from build123d import *

# Parameters (mm, degrees)
PAD_DEPTH            = 70
SKETCH001_W          = 11.887794
SKETCH001_H          = 46.78
POCKET_DEPTH         = 70.001
POCKET001_DEPTH      = 30
SKETCH003_R          = 2.5
POCKET002_DEPTH      = 40.001
SKETCH004_W          = 17
SKETCH004_H          = 23.314381
POCKET003_DEPTH      = 40.001
SKETCH005_W          = 35
SKETCH005_H          = 57.974789
POCKET004_DEPTH      = 26
SKETCH006_W          = 45.255611
SKETCH006_H          = 30.428207
POCKET005_DEPTH      = 28
POCKET005_DEPTH_BACK = -100
SKETCH007_W          = 26.242121
SKETCH007_H          = 29.741062
POCKET006_DEPTH      = 45
SKETCH008_W          = 15.625622
SKETCH008_H          = 14.392597
SKETCH008_W_2        = 24.610352
SKETCH008_H_2        = 31.67345
POCKET007_DEPTH      = 45
SKETCH009_R          = 2.5
POCKET008_DEPTH      = 13
SKETCH010_R          = 1.6
POCKET009_DEPTH      = 5
SKETCH014_W          = 10
SKETCH014_H          = 15
PAD001_DEPTH         = 23
SKETCH015_W          = 11
SKETCH015_H          = 38.184422
SKETCH015_W_2        = 19.881198
SKETCH015_H_2        = 10
PAD002_DEPTH         = 8
SKETCH013_R          = 2.5
POCKET010_DEPTH      = 17
SKETCH011_R          = 2.5
POCKET011_DEPTH      = 15
PAD003_DEPTH         = 5
SKETCH017_R          = 3
POCKET012_DEPTH      = 2
FILLET_R             = 1
FILLET001_R          = 7
FILLET002_R          = 1
FILLET003_R          = 1
FILLET004_R          = 2
FILLET005_R          = 2
FILLET006_R          = 18


with BuildPart() as part:
    # Sketch → Pad (new body)
    with BuildSketch(Plane.XY):
        Polygon((0, 0), (45, 0), (45, -50), (-28, -50), (-28, 0), align=None)
    extrude(amount=PAD_DEPTH)

    # Sketch001 (on Face7 of Pad) → Pocket (cut, through all)
    with BuildSketch(Plane.XY.offset(70)):
        with Locations((34.056103, -28.39)):
            Rectangle(SKETCH001_W, SKETCH001_H)
    extrude(amount=-POCKET_DEPTH, mode=Mode.SUBTRACT)

    # Sketch002 (on Face5 of Pocket) → Pocket001 (cut)
    with BuildSketch(Plane.XY.offset(70)):
        Polygon((30, -5), (30, -65.096024), (-40.783405, -65.096024), (-40.783405, 12.994774), (20, 12.994774), (20, -5), align=None)
    extrude(amount=-POCKET001_DEPTH, mode=Mode.SUBTRACT)

    # Sketch003 (on Face6 of Pocket001) → Pocket002 (cut, through all)
    with BuildSketch(Plane.XY.offset(40)):
        with Locations((-22, -40)):
            Circle(SKETCH003_R)
        with Locations((22, -40)):
            Circle(SKETCH003_R)
    extrude(amount=-POCKET002_DEPTH, mode=Mode.SUBTRACT)

    # Sketch004 (on Face6 of Pocket002) → Pocket003 (cut, through all)
    with BuildSketch(Plane.XY.offset(40)):
        with Locations((0, -43.65719)):
            Rectangle(SKETCH004_W, SKETCH004_H)
    extrude(amount=-POCKET003_DEPTH, mode=Mode.SUBTRACT)

    # Sketch005 (on Face13 of Pocket003) → Pocket004 (cut)
    with BuildSketch(Plane.XZ.offset(50)):
        with Locations((0, 7.512606)):
            Rectangle(SKETCH005_W, SKETCH005_H)
    extrude(amount=-POCKET004_DEPTH, mode=Mode.SUBTRACT)

    # Sketch006 (on Face11 of Pocket004) → Pocket005 (cut, two sides)
    with BuildSketch(Plane.XZ.offset(24)) as pocket005_sk:
        with Locations((-10.127806, 6.785896)):
            Rectangle(SKETCH006_W, SKETCH006_H)
    extrude(amount=-POCKET005_DEPTH, mode=Mode.SUBTRACT)
    extrude(pocket005_sk.sketch, amount=-POCKET005_DEPTH_BACK, mode=Mode.SUBTRACT)

    # Sketch007 (on Face12 of Pocket005) → Pocket006 (cut)
    with BuildSketch(Plane.XZ.offset(50)):
        with Locations((20.733142, 3.968048)):
            Rectangle(SKETCH007_W, SKETCH007_H)
    extrude(amount=-POCKET006_DEPTH, mode=Mode.SUBTRACT)

    # Sketch008 (on Face14 of Pocket006) → Pocket007 (cut)
    with BuildSketch(Plane.XZ.offset(50)):
        with Locations((42.909006, 69.196298)):
            Rectangle(SKETCH008_W, SKETCH008_H)
        with Locations((46.359665, 3.163275)):
            Rectangle(SKETCH008_W_2, SKETCH008_H_2)
    extrude(amount=-POCKET007_DEPTH, mode=Mode.SUBTRACT)

    # Sketch009 (on Face3 of Pocket007) → Pocket008 (cut)
    with BuildSketch(Plane.YZ.offset(45)):
        with Locations((-44, 55)):
            Circle(SKETCH009_R)
        with Locations((-13, 24)):
            Circle(SKETCH009_R)
        with Locations((-13, 55)):
            Circle(SKETCH009_R)
        with Locations((-44, 24)):
            Circle(SKETCH009_R)
    extrude(amount=-POCKET008_DEPTH, mode=Mode.SUBTRACT)

    # Sketch010 (on Face1 of Pocket008) → Pocket009 (cut)
    with BuildSketch(Plane(origin=(0, 0, 0), x_dir=(-1, 0, 0), z_dir=(0, 1, 0))):
        with Locations((-33, 5)):
            Circle(SKETCH010_R)
        with Locations((-40, 65)):
            Circle(SKETCH010_R)
        with Locations((-26, 65)):
            Circle(SKETCH010_R)
    extrude(amount=-POCKET009_DEPTH, mode=Mode.SUBTRACT)

    # Sketch014 (on Face4 of Pocket009) → Pad001 (join)
    with BuildSketch(Plane.YZ.offset(45)):
        with Locations((-30, 32.5)):
            Rectangle(SKETCH014_W, SKETCH014_H)
    extrude(amount=-PAD001_DEPTH)

    # Sketch015 (on Face29 of Pad001) → Pad002 (join)
    with BuildSketch(Plane(origin=(-28, 0, 0), x_dir=(0, -1, 0), z_dir=(-1, 0, 0))):
        with Locations((13.5, 54.907789)):
            Rectangle(SKETCH015_W, SKETCH015_H)
        with Locations((52.059401, 30)):
            Rectangle(SKETCH015_W_2, SKETCH015_H_2)
    extrude(amount=-PAD002_DEPTH)

    # Sketch013 (on Face19 of Pad002) → Pocket010 (cut)
    with BuildSketch(Plane.XZ.offset(24)):
        with Locations((-7, 30.5)):
            Circle(SKETCH013_R)
        with Locations((7, 30.5)):
            Circle(SKETCH013_R)
    extrude(amount=-POCKET010_DEPTH, mode=Mode.SUBTRACT)

    # Sketch011 (on Face29 of Pad002) → Pocket011 (cut)
    with BuildSketch(Plane(origin=(-28, 0, 0), x_dir=(0, -1, 0), z_dir=(-1, 0, 0))):
        with Locations((56.5, 30)):
            Circle(SKETCH011_R)
        with Locations((13, 68.5)):
            Circle(SKETCH011_R)
    extrude(amount=-POCKET011_DEPTH, mode=Mode.SUBTRACT)

    # Sketch016 (on Face1 of Pocket011) → Pad003 (join)
    with BuildSketch(Plane(origin=(0, 0, 0), x_dir=(-1, 0, 0), z_dir=(0, 1, 0))):
        Polygon((-12.5, 0), (5, 22), (-15.71, 22), align=None)
    extrude(amount=-PAD003_DEPTH)

    # Sketch017 (on Face28 of Pad003) → Pocket012 (cut)
    with BuildSketch(Plane.XZ.offset(5)):
        with Locations((26, 65)):
            Circle(SKETCH017_R)
        with Locations((33, 5)):
            Circle(SKETCH017_R)
        with Locations((40, 65)):
            Circle(SKETCH017_R)
    extrude(amount=-POCKET012_DEPTH, mode=Mode.SUBTRACT)

    # Fillet
    fillet_edges = [part.edges().sort_by_distance(p)[0] for p in [
        (-28, -25, 22),
    ]]
    fillet(fillet_edges, radius=FILLET_R)

    # Fillet001
    fillet001_edges = [part.edges().sort_by_distance(p)[0] for p in [
        (45, -2.5, 0),
    ]]
    fillet(fillet001_edges, radius=FILLET001_R)

    # Fillet002
    fillet002_edges = [part.edges().sort_by_distance(p)[0] for p in [
        (45, -27.5, 19),
    ]]
    fillet(fillet002_edges, radius=FILLET002_R)

    # Fillet003
    fillet003_edges = [part.edges().sort_by_distance(p)[0] for p in [
        (45, -27.5, 62),
    ]]
    fillet(fillet003_edges, radius=FILLET003_R)

    # Fillet004
    fillet004_edges = [part.edges().sort_by_distance(p)[0] for p in [
        (45, -2.5, 70),
    ]]
    fillet(fillet004_edges, radius=FILLET004_R)

    # Fillet005
    fillet005_edges = [part.edges().sort_by_distance(p)[0] for p in [
        (20, -2.5, 70),
    ]]
    fillet(fillet005_edges, radius=FILLET005_R)

    # Fillet006
    fillet006_edges = [part.edges().sort_by_distance(p)[0] for p in [
        (20, -2.5, 40),
    ]]
    fillet(fillet006_edges, radius=FILLET006_R)


solid = part.part
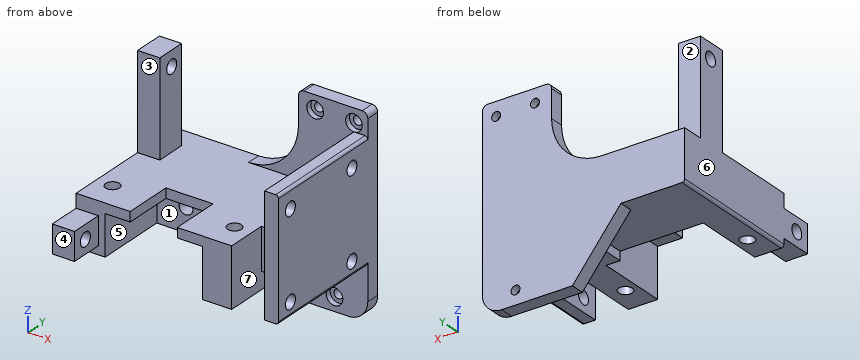
Build history of the part. All positions in model axes, mm. Face numbers are marked on the shaded views. A direction names the side the tool comes from. Coordinates: 2 decimals unless noted, no trailing zeros. Order: outer loops, then holes, each group sorted by start corner. A loop starts at its lowest first (then second) coordinate and runs counter-clockwise, first axis right, second up. Notation, with made-up numbers: (82.25, 3) - (88.25, 3) arc R12 cw to (88.25, 21) - close; hole circle Ø6 at (49, -31). An arc over 180 degrees is marked (long way). Write item = value, one per line. Start each with the question number.
1) Flat gauge pins, fed straight in: pin 1 Ø2 at (y, z) = (-54.5, 28) entering from +X; pin 2 Ø5 at (x, z) = (33, 5) entering from -Y; pin 3 Ø3.5 at (x, z) = (33.5, 33.5) entering from -Y; pin 4 Ø6 at (x, z) = (15, 61.5) entering from -Y. Where does each tip first touch, or does it go through?
2) Saw through at A-A on x = -22. Write the cut outline in (y, z).
3) Saw through at B-B on y = -56.5. Write the cut outline in (x, z), then the cut area to 3 significant figures.
4) Saw through at C-C on z = 24. Write the cut outline in (x, y), then the cut area to 3 significant figures.
5) Wall check: line 1 along Z through (x, y) = (26, -1.5); line 2 along X through (y, z) = (-11, 49); line 3 along X through (y, z) = (-27.5, 36). Give the ranges that are in metal, low to high. Write a range as from..to.
6) Two-plate mould, pull along X, no slides. Class the marked faces 4, 5, 6 and 7: pulls with the +X half, pulls with the -X half, needs draft (parallel to the pull), parting line crosses it, or undercut.
7) Saw through at D-D on x = 33. Write the cut outline in (y, z).
8) 3-axis set-ups, long thin cutter, end or side, ignore diameter. For the marked faces 1, 2 and 3: which of +Z, -Z, +X, -X, +Y, -Y reach the whole face in a straight line?
From the geometry:
q1.pin_1 = -20
q1.pin_2 = -3
q1.pin_3 = -35
q1.pin_4 = through
q2.outline = (-62, 25) - (-50, 25) - (-50, 22) - (-42.5, 22) - (-42.5, 25) - (-42.12, 25) - (-42.12, 35) - (-42.5, 35) - (-42.5, 40) - (-50, 40) - (-50, 35) - (-62, 35) - close; (-37.5, 22) - (0, 22) - (0, 40) - (-8, 40) - (-8, 74) - (-19, 74) - (-19, 40) - (-37.5, 40) - close; hole circle Ø5 at (-56.5, 30); hole circle Ø5 at (-13, 68.5)
q3.outline = (-28, 25) - (-20, 25) - (-20, 27.5) - (-28, 27.5) - close; (-28, 32.5) - (-20, 32.5) - (-20, 35) - (-28, 35) - close
q3.area = 40.0 mm^2
q4.outline = (-28, -50) - (-17.5, -50) - (-17.5, -24) - (17.5, -24) - (17.5, -50) - (28.11, -50) - (28.11, -5) - (40, -5) - (40, -10.5) - (45, -10.5) - (45, 0) - (-28, 0) - close; (40, -50) - (45, -50) - (45, -46.5) - (40, -46.5) - close; (40, -41.5) - (45, -41.5) - (45, -15.5) - (40, -15.5) - close; hole circle Ø5 at (-22, -40); hole circle Ø5 at (22, -40)
q4.area = 2,120 mm^2
q5.line_1 = 0..63.4, 66.6..70
q5.line_2 = -28..-20, 40..45
q5.line_3 = -28..-17.5, 17.5..45
q6.face_4 = needs draft
q6.face_5 = undercut
q6.face_6 = pulls with the -X half
q6.face_7 = undercut
q7.outline = (-35, 25) - (-25, 25) - (-25, 40) - (-35, 40) - close; (-5, 0) - (0, 0) - (0, 3.4) - (-3, 3.4) - (-3, 2) - (-5, 2) - close; (-5, 8) - (-3, 8) - (-3, 6.6) - (0, 6.6) - (0, 70) - (-5, 70) - close
q8.face_1 = -Z, -Y
q8.face_2 = +Z, -X, +Y
q8.face_3 = +Z, -X, -Y
